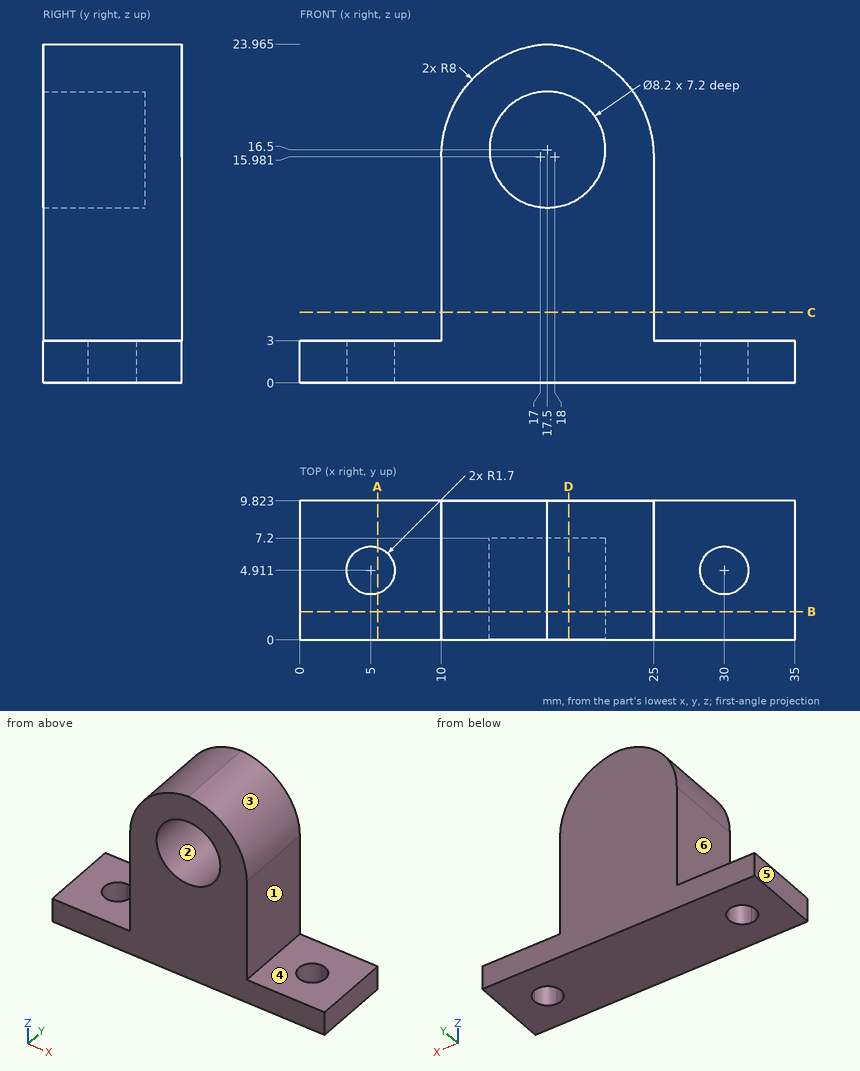
Input: dimensioned drawing with shaded views. Units: mm. Origin: part minimum x, y, z. A direction names the side the tool comes from. Round coordinates to 2 decimals unless told otherwise and drop trailing zeros. Loops run counter-clockwise (first coordinate to the right, second up) from the corner with the lowest first, then second, coordinate; pieces in that order, holes last. Notation, with made-up numbers: M 75.25,20.25 L 113.25,20.25 A9 cw 113.25,31.25 Z; hole C -37.75,-11.75 d10. An arc over 180 degrees is marked long. One line per question, with ' | ' between items.
(1) Cut plane A-A on x = 5.5. Return the cut outline in (y, z).
Check result:
outline: M 0,0 L 3.29,0 L 3.29,3 L 0,3 Z; M 6.54,0 L 9.82,0 L 9.82,3 L 6.54,3 Z
(2) Access query for the marked faces 4, 5 and 6. Directions: +Z, -Z, +X, -X, +Y, -Y. A direction counts if a zero-diameter tool reaches every point of the face in a straight line with its end or side. Return the directions, or none.
Check result:
face 4: +Z, +X, +Y, -Y | face 5: +Z, -Z, -X, +Y, -Y | face 6: +Z, -X, +Y, -Y
(3) Cut plane C-C on z = 5. Return the cut outline in (x, y).
Check result:
outline: M 10,0 L 25,0 L 25,9.82 L 10,9.82 Z
(4) Contact query for flat-ended pins moving along their axis: P1, Ø5, axis at y = 6, z = 11.5, coming from the -X side; P2, Ø1.5, axis at y = 1.5, z = 17.5, coming from the +X side; P3, Ø3, axis at x = 28.5, y = 2.5, coming from the +Z side. Output: stop coordinate, or through.
Check result:
P1: stops at x = 10 | P2: stops at x = 24.96 | P3: stops at z = 3
(5) Cut plane B-B on y = 2. Return the cut outline in (x, z) (1 decimal).
Check result:
outline: M 0,0 L 35,0 L 35,3 L 25,3 L 25,16 A8 ccw 17.5,24 A8 ccw 10,16 L 10,3 L 0,3 Z; hole C 17.5,16.5 d8.2
(6) Material intervals for line 1 along X through (y, z) = (5.75, 4.25); line 2 along X through (y, z) = (5.25, 2) (1 decimal); line 3 along X through (y, z) = (4, 12.75) (1 decimal), sorted ascending. Write a range as from..to.
Check result:
line 1: x = 10..25 | line 2: x = 0..3.3, 6.7..28.3, 31.7..35 | line 3: x = 10..15.8, 19.2..25
(7) Cut plane D-D on x = 19. Return the cut outline in (y, z), plus the area to 3 significant figures.
Check result:
outline: M 0,0 L 9.82,0 L 9.82,23.73 L 0,23.73 L 0,20.32 L 7.2,20.32 L 7.2,12.68 L 0,12.68 Z | area: 178 mm2
(8) Pull-direction query (Z, two-part tool) for the marked faces 1, 2 and 3; classes: +Z half, -Z half, draft (parallel to the pull), parting line (faces both ways), or undercut.
Check result:
face 1: draft | face 2: undercut | face 3: +Z half
